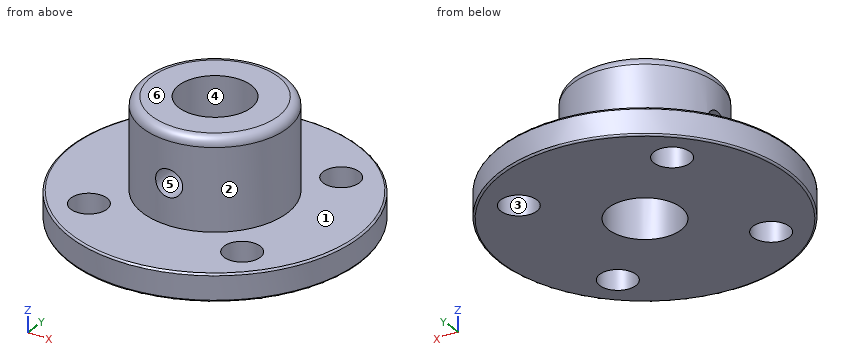
from build123d import *

# Parameters (mm, degrees)
SKETCH1_R           = 16
BOSS_EXTRUDE1_DEPTH = 3
SKETCH2_R           = 8
BOSS_EXTRUDE2_DEPTH = 10
SKETCH3_R           = 4
CUT_EXTRUDE1_DEPTH  = 14
SKETCH4_R           = 2
CUT_EXTRUDE2_DEPTH  = 4
FILLET1_R           = 1
SKETCH5_R           = 1.5
CUT_EXTRUDE3_DEPTH  = 9
SKETCH6_R           = 1.5
CUT_EXTRUDE4_DEPTH  = 9
FILLET2_R           = 0.2


with BuildPart() as part:
    # Sketch1 → Boss-Extrude1 (new body)
    with BuildSketch(Plane.XY):
        Circle(SKETCH1_R)
    extrude(amount=BOSS_EXTRUDE1_DEPTH)

    # Sketch2 → Boss-Extrude2 (add)
    with BuildSketch(Plane.XY.offset(3)):
        Circle(SKETCH2_R)
    extrude(amount=BOSS_EXTRUDE2_DEPTH)

    # Sketch3 → Cut-Extrude1 (cut, through all)
    with BuildSketch(Plane.XY.offset(13)):
        Circle(SKETCH3_R)
    extrude(amount=-CUT_EXTRUDE1_DEPTH, mode=Mode.SUBTRACT)

    # Sketch4 → Cut-Extrude2 (cut, through all)
    with BuildSketch(Plane.XY.offset(3)):
        with Locations((-8.485281374, 8.485281374)):
            Circle(SKETCH4_R)
        with Locations((8.485281374, 8.485281374)):
            Circle(SKETCH4_R)
        with Locations((8.485281374, -8.485281374)):
            Circle(SKETCH4_R)
        with Locations((-8.485281374, -8.485281374)):
            Circle(SKETCH4_R)
    extrude(amount=-CUT_EXTRUDE2_DEPTH, mode=Mode.SUBTRACT)

    # Fillet1
    fillet1_edges = [part.edges().sort_by_distance(p)[0] for p in [
        (-8, 0, 13),
    ]]
    fillet(fillet1_edges, radius=FILLET1_R)

    # Sketch5 → Cut-Extrude3 (cut)
    with BuildSketch(Plane(origin=(0, 0, 0), x_dir=(0, 0, -1), z_dir=(1, 0, 0))):
        with Locations((-7.5, 0)):
            Circle(SKETCH5_R)
    extrude(amount=-CUT_EXTRUDE3_DEPTH, mode=Mode.SUBTRACT)

    # Sketch6 → Cut-Extrude4 (cut)
    with BuildSketch(Plane(origin=(0, 0, 0), x_dir=(1, 0, 0), z_dir=(0, 1, 0))):
        with Locations((0, -7.5)):
            Circle(SKETCH6_R)
    extrude(amount=-CUT_EXTRUDE4_DEPTH, mode=Mode.SUBTRACT)

    # Fillet2
    fillet2_edges = [part.edges().sort_by_distance(p)[0] for p in [
        (-16, 0, 0),
        (-16, 0, 3),
    ]]
    fillet(fillet2_edges, radius=FILLET2_R)


solid = part.part
Work out the finished part from the listing and answer in its coordinate system (mm). Face numbers are marked on the shaded views. A direction names the side the tool comes from. Round coordinates to 2 decimals unless told otherwise and drop trailing zeros. Loops run counter-clockwise (first coordinate to the right, second up) from the corner with the lowest first, then second, coordinate; pieces in that order, holes last. Notation, with made-up numbers: M 60.5,-36.5 L 100.5,-36.5 A28 ccw 100.5,-16.5 Z; hole C 36,-35 d4. An arc over 180 degrees is marked long. One line per question, with ' | ' between items. Start each with the question number.
(1) Flat-ended cylindrical pins translate along their axes: pin 1 Ø2.5 at (y, z) = (0, 7.5) entering from +X; pin 2 Ø2.5 at (x, z) = (0, 7.5) entering from +Y; pin 3 Ø1 at (x, z) = (-2, 6.5) entering from -Y; pin 4 Ø3.5 at (x, y) = (8.49, 8.49) entering from +Z (3 decimals). Find the tip coordinate at first contact, or state that the pin passes through.
(2) For a pull along X with two mould halves and no side action, classify the marked faces 1, 2, 3 and 4 as released by +X, released by -X, zero draft, split by the parting line, or undercut.
(3) A tool of negligible diameter and unlimited length cuts with its end or side. For the marked faces 5 and 6, from which of +Z, -Z, +X, -X, +Y, -Y can it reach the whole face along a straight path? Write none if from no direction.
(4) Find the intervals of material crossed by line 1 (Z direction, x = 0, y = -4.9); line 2 (X direction, y = 3.5, z = 8); line 3 (Y direction, x = -4.5, z = 7.75), in increasing order.
(5) A cutting plane is placed at A-A on x = 0. Write down the section's boundary in (y, z), plus the area to 3 significant figures.
(6) A cutting plane is placed at D-D on z = 11.5. Write down the section's boundary in (x, y), plus the area to 3 significant figures.
(7) A cutting plane is placed at C-C on z = 7.5. Write down the section's boundary in (x, y).
Geometry check:
1) pin 1: stops at x = 8 | pin 2: stops at y = 8 | pin 3: stops at y = -7.86 | pin 4: passes through
2) face 1: zero draft | face 2: split by the parting line | face 3: undercut | face 4: undercut
3) face 5: -Y | face 6: +Z, +X, -X, +Y, -Y
4) line 1: z = 0 to 6, 9 to 13 | line 2: x = -7.19 to -1.94, 1.94 to 7.19 | line 3: y = -6.61 to -1.48, 1.48 to 6.61
5) outline: M -16,0.2 A0.2 ccw -15.8,0 L -4,0 L -4,6 L -8,6 L -8,3 L -15.8,3 A0.2 ccw -16,2.8 Z; M -8,9 L -4,9 L -4,13 L -7,13 A1 ccw -8,12 Z; M 4,0 L 15.8,0 A0.2 ccw 16,0.2 L 16,2.8 A0.2 ccw 15.8,3 L 8,3 L 8,12 A1 ccw 7,13 L 4,13 Z | area: 140 mm²
6) outline: C 0,0 d16; hole C 0,0 d8 | area: 151 mm²
7) outline: M -7.86,-1.5 A8 ccw -1.5,-7.86 L -1.5,-3.71 A4 cw -3.71,-1.5 Z; M -7.86,1.5 L -3.71,1.5 A4 cw long 1.5,-3.71 L 1.5,-7.86 A8 ccw long Z
